Input: part model. Units: mm. Frame: model coordinates. Give positions to 0.01 mm unless a question says otherwise; leave off trailing zeros. Order: outer loops, then holes, each group sorted by start corner. A loop starts at its lowest first (then second) coordinate and runs counter-clockwise, first axis right, second up.
```python
from build123d import *

# Parameters (mm, degrees)
SKETCH005_R      = 5
SKETCH005_R_2    = 2.105463
EXTRUDE004_DEPTH = 9
SKETCH004_R      = 2.2
EXTRUDE003_DEPTH = 5


with BuildPart() as psu_one_hole_extrude:
    # Sketch005 → Extrude004 (new body)
    with BuildSketch(Plane.XY):
        with Locations((-39.96372, 49.017672)):
            Circle(SKETCH005_R)
        with Locations((-39.959132, 49.020638)):
            Circle(SKETCH005_R_2, mode=Mode.SUBTRACT)
    extrude(amount=EXTRUDE004_DEPTH)


with BuildPart() as psu_two_hole_tab_fusion:
    # Sketch004 → Extrude003 (new body)
    with BuildSketch(Plane.XY):
        with BuildLine():
            Line((-39.96372, 54.017672), (-19.96372, 54.017672))
            ThreePointArc((-19.96372, 44.017672), (-14.96372, 49.017672), (-19.96372, 54.017672))
            Line((-39.96372, 44.017672), (-19.96372, 44.017672))
            ThreePointArc((-39.96372, 54.017672), (-44.96372, 49.017672), (-39.96372, 44.017672))
        make_face()
        with Locations((-39.96372, 49.017672)):
            Circle(SKETCH004_R, mode=Mode.SUBTRACT)
        with Locations((-19.96372, 49.017672)):
            Circle(SKETCH004_R, mode=Mode.SUBTRACT)
    extrude(amount=EXTRUDE003_DEPTH)

    # Fusion008: union psu one hole extrude
    add(psu_one_hole_extrude.part)


solid = psu_two_hole_tab_fusion.part
```
1) Pull-direction query (X, two-part tool) for faces 1 (the face through (-27, 49, 5)), 2 (the face through (-44.96, 49.24, 5.44)), 3 (the face through (-38.99, 47.15, 4.44)); classes: pulls with the +X half, pulls with the -X half, needs draft (parallel to the pull), parting line crosses it, or undercut.
2) Cut plane A-A (y = 47.5). Return the cut outline in (x, z).
3) Line query: probe 1 along X at (y, z) = (49, 8); probe 2 along X at (y, z) = (48.75, 1.5); probe 3 along Z at (x, y) = (-32, 45.5). Output: solid intervals per line, ascending.
4) Cut plane D-D (x = -36). Return the cut outline in (y, z), then the cut area to 3 significant figures.
5) Cut plane C-C (z = 0.5). Return the cut outline in (x, y), then the cut area to 3 significant figures.
6) Cut plane B-B (x = -19.5). Return the cut outline in (y, z).
7) First-contact query: P1, Ø1.5, axis at y = 46, z = 1.5, coming from the -X side; P2, Ø1, axis at y = 46.5, z = 2, coming from the -X side; P3, Ø2, axis at y = 45, z = 3.5, coming from the -X side. Flat tips, straight axial feed; report the tip coordinate or a pass-through.
Geometry says:
1. face 1: needs draft
1. face 2: parting line crosses it
1. face 3: undercut
2. outline: (-44.73, 0) - (-41.42, 0) - (-41.42, 9) - (-44.73, 9) - close; (-38.5, 0) - (-21.56, 0) - (-21.56, 5) - (-35.2, 5) - (-35.2, 9) - (-38.5, 9) - close; (-18.37, 0) - (-15.2, 0) - (-15.2, 5) - (-18.37, 5) - close
3. probe 1: x = -44.96 to -42.06, -37.85 to -34.96
3. probe 2: x = -44.96 to -42.05, -37.87 to -22.15, -17.78 to -14.97
3. probe 3: z = 0 to 5
4. outline: (44.02, 0) - (54.02, 0) - (54.02, 5) - (52.07, 5) - (52.07, 9) - (45.97, 9) - (45.97, 5) - (44.02, 5) - close
4. area: 74.4 mm2
5. outline: (-39.96, 44.02) - (-19.96, 44.02) arc R5 ccw to (-19.96, 54.02) - (-39.96, 54.02) arc R5 ccw to start; hole circle Ø4.21 at (-39.96, 49.02); hole circle Ø4.4 at (-19.96, 49.02)
5. area: 249 mm2
6. outline: (44.04, 0) - (46.87, 0) - (46.87, 5) - (44.04, 5) - close; (51.17, 0) - (54, 0) - (54, 5) - (51.17, 5) - close
7. P1: stops at x = -44.42
7. P2: stops at x = -44.54
7. P3: stops at x = -43.95
